Read the model definition and answer for the solid it produces. Units are mm, in the model's axes. A direction names the side the tool comes from. Give positions to 0.01 mm unless a question says otherwise; leave off trailing zeros. Order: outer loops, then holes, each group sorted by start corner. A loop starts at its lowest first (then second) coordinate and runs counter-clockwise, first axis right, second up. Notation, with made-up numbers: (16, -10.75) - (54, -10.75) arc R12 ccw to (54, 12.25) - close; hole circle Ø5 at (81.5, 39). An arc over 180 degrees is marked (long way). Return JSON: item names as keys, results as strings.
```python
from build123d import *

# Parameters (mm, degrees)
F1_DEPTH = 20
F2_R     = 2.25
F3_DEPTH = 39.001


# Not quite as in the source:
# - a pattern or mirror of a feature is missing from the dataset's text; its kind, count and spacing are read off the source's solid


with BuildPart() as f1:
    # F0 (on Top) → F1 (new body)
    with BuildSketch(Plane.XY):
        Polygon((0, 26.5), (0, 0), (4, 0), (4, 22.5), (39, 22.5), (39, 41.5), (35, 41.5), (35, 26.5), align=None)
        Polygon((4, 0), (0, 0), (0, -26.5), (35, -26.5), (35, -41.5), (39, -41.5), (39, -22.5), (4, -22.5), align=None)
    extrude(amount=F1_DEPTH)

    # F2 (on Right) → F3 (cut, through all)
    with BuildSketch(Plane.YZ):
        with Locations((34.5, 10)):
            Circle(F2_R)
    f3 = extrude(amount=F3_DEPTH, mode=Mode.SUBTRACT)

    # F3_copies: F3 across plane
    add(f3.mirror(Plane(origin=(0, 0, 0), x_dir=(0, 0, -1), z_dir=(0, -1, 0))), mode=Mode.SUBTRACT)


solid = f1.part
```
Q1. Determine the mould class of faces 4 (the flat face through (35, -32, 10)), 5 (the flat face through (22, -22.5, 10)), 6 (the flat face through (17, -26.5, 10)), 7 (the flat face through (4, 0, 10)) for opening direction Y: released by +Y, released by -Y, zero draft, split by the parting line, or undercut.
Values:
{"face 4": "zero draft", "face 5": "undercut", "face 6": "released by -Y", "face 7": "undercut"}
Q2. Consider L1, parallel to Z at x = 37.35, y = 34.5; L2, parallel to Y at x = 18.5, z = 3.75; L3, parallel to X at y = -22, z = 8. Determine where each line is inside the solid, lowest interval first.
Values:
{"L1": "z = 0 to 7.75, 12.25 to 20", "L2": "y = -26.5 to -22.5, 22.5 to 26.5", "L3": "x = 0 to 4"}
Q3. For faces 1 (the flat face through (3.5, -2.9, 20)), 2 (the flat face through (21, 22.5, 10)), 3 (the flat face through (35, 34.1, 7.6)), determine the directions among +Z, -Z, +X, -X, +Y, -Y from which every point of the face is accessible in a straight line to the end or side of a thin tool.
Values:
{"face 1": "+Z, +X, -X, +Y, -Y", "face 2": "+Z, -Z, +X", "face 3": "+Z, -Z, -X, +Y"}
Q4. A cutting plane is placed at D-D (y = -18). Write down the section's boundary in (x, z), and give its area (3 significant figures).
Values:
{"outline": "(0, 0) - (4, 0) - (4, 20) - (0, 20) - close", "area": "80.0 mm²"}
Q5. A cutting plane is placed at B-B (y = -34.5). Write down the section's boundary in (x, z).
Values:
{"outline": "(35, 0) - (39, 0) - (39, 7.75) - (35, 7.75) - close; (35, 12.25) - (39, 12.25) - (39, 20) - (35, 20) - close"}
Q6. Given pin 1 (7.5 mm diameter, centred on y = -35.5, z = 13, fed in from -X); pin 2 (6 mm diameter, centred on x = 20.5, z = 14.5, fed in from -Y); pin 3 (2 mm diameter, centred on y = -15, z = 14.5, fed in from -X); pin 4 (10 mm diameter, centred on x = 22, z = 6.5, fed in from +Y), each flat-ended and moving along its own axis, determine where each tip first touches the part or whether it passes through.
Values:
{"pin 1": "stops at x = 35", "pin 2": "stops at y = -26.5", "pin 3": "stops at x = 0", "pin 4": "stops at y = 26.5"}
Q7. A cutting plane is placed at C-C (z = 2). Write down the section's boundary in (x, y).
Values:
{"outline": "(0, -26.5) - (35, -26.5) - (35, -41.5) - (39, -41.5) - (39, -22.5) - (4, -22.5) - (4, 22.5) - (39, 22.5) - (39, 41.5) - (35, 41.5) - (35, 26.5) - (0, 26.5) - close"}
Q8. A cutting plane is placed at A-A (x = 5). Write down the section's boundary in (y, z).
Values:
{"outline": "(-26.5, 0) - (-22.5, 0) - (-22.5, 20) - (-26.5, 20) - close; (22.5, 0) - (26.5, 0) - (26.5, 20) - (22.5, 20) - close"}
